Here's how the part is built. I have some questions about the finished solid (model axes, mm). A direction names the side the tool comes from. Round coordinates to 2 decimals unless told otherwise and drop trailing zeros. Loops run counter-clockwise (first coordinate to the right, second up) from the corner with the lowest first, then second, coordinate; pieces in that order, holes last. Notation, with made-up numbers: (76.25, 74) -> (102.25, 74) arc R24 ccw to (102.25, 89) -> close; hole circle Ø10 at (-11.75, 24.25). An arc over 180 degrees is marked (long way). Use one line per item in the form item = value. Start each with the question number.
Item 1: Thinking about a two-plate mould opening in X: for faces 1 (the face through (-20.345, 2.028, 21.979)), 2 (the face through (27.8, 11, 0)), 3 (the face through (0, 0, 0)), which applies, released by +X, released by -X, zero draft, split by the parting line, or undercut?
Item 2: If I drill on L1, parallel to X at y = 2.4, z = 21.5; L2, parallel to Z at x = 21, y = 1, over which ranges is the centre line in solid material (lowest first)? Write a range as [from, to].
Item 3: I'm going to push flat-ended pins straight in: pin 1 Ø2 at (x, z) = (21.5, 21.5) entering from -Y; pin 2 Ø2 at (x, z) = (21.5, -21.5) entering from +Y; pin 3 Ø12 at (y, z) = (33, 10.5) entering from -X. Where does each tip first touch, or does it pass through?
Item 4: If we section it at A-A (y = 30.5): Write out the boundary of the cut face in (x, z).
Item 5: For faces 4 (the face through (-26.37, 11.71, 26.3)), 5 (the face through (-27, 23.1, 6)), 6 (the face through (-22, 4, -22)), which set-ups out of +Z, -Z, +X, -X, +Y, -Y let a thin tool reach every point of the face, with its end or its side?
```python
from build123d import *

# Parameters (mm, degrees)
SKETCH_2_W          = 55.6
SKETCH_2_H          = 55.6
EXTRUDE_1_DEPTH     = 23.1
SKETCH_3_R          = 27.5
EXTRUDE_2_DEPTH     = 18.2
HOLE_WIZARD_1_D     = 2.5
HOLE_WIZARD_1_DEPTH = 4
FILLET_1_R          = 5
FILLET_2_R          = 2


with BuildPart() as part:
    # 草图2 → 凸台-拉伸1 (new body)
    with BuildSketch(Plane(origin=(0, 0, 0), x_dir=(1, 0, 0), z_dir=(0, 1, 0))):
        Rectangle(SKETCH_2_W, SKETCH_2_H)
    extrude(amount=EXTRUDE_1_DEPTH)

    # 草图3 → 凸台-拉伸2 (add)
    with BuildSketch(Plane(origin=(0, 23.1, 0), x_dir=(1, 0, 0), z_dir=(0, 1, 0))):
        with Locations(Location((0, 0, 0), (0, 0, 270))):
            Circle(SKETCH_3_R)
    extrude(amount=EXTRUDE_2_DEPTH)

    # 孔1
    with Locations(Plane(origin=(0, 0, 0), x_dir=(-1, 0, 0), z_dir=(0, -1, 0))):
        with Locations((-21.5, 21.5), (21.5, 21.5), (21.5, -21.5), (-21.5, -21.5)):
            Hole(HOLE_WIZARD_1_D / 2, depth=HOLE_WIZARD_1_DEPTH)

    # 圆角1
    fillet_1_edges = [part.edges().sort_by_distance(p)[0] for p in [
        (27.8, 11.55, 27.8),
        (-27.8, 11.55, 27.8),
        (-27.8, 11.55, -27.8),
        (27.8, 11.55, -27.8),
    ]]
    fillet(fillet_1_edges, radius=FILLET_1_R)

    # 圆角2
    fillet_2_edges = [part.edges().sort_by_distance(p)[0] for p in [
        (0, 41.3, -27.5),
    ]]
    fillet(fillet_2_edges, radius=FILLET_2_R)


solid = part.part
```
Values found:
q1.face_1 = undercut
q1.face_2 = released by +X
q1.face_3 = zero draft
q2.L1 = [-27.8, -22.75], [-20.25, 20.25], [22.75, 27.8]
q2.L2 = [-27.8, -22.65], [-20.35, 20.35], [22.65, 27.8]
q3.pin_1 = 4
q3.pin_2 = 23.1
q3.pin_3 = -27.13
q4.outline = circle Ø55 at (0, 0)
q5.face_4 = +Z, -X, +Y, -Y
q5.face_5 = +Y
q5.face_6 = -Y
